```python
from build123d import *

# Parameters (mm, degrees)
FILLET1_R           = 6.35
SKETCH11_R          = 28.575
BOSS_EXTRUDE2_DEPTH = 1143
FILLET2_R           = 6.35
SCALE1_SCALE        = 0.5
SCALE2_SCALE        = 0.25


with BuildPart() as part:
    # Sketch7 → Revolve4 (revolve)
    with BuildSketch(Plane(origin=(0, 0, 0), x_dir=(1, 0, 0), z_dir=(0, 1, 0))):
        with BuildLine():
            Line((-190.055393274, 59.537811837), (0, 46.530218381))
            Line((0, 46.530218381), (0, 0))
            Line((0, 0), (-253.807316321, 0))
            ThreePointArc((-253.807316321, 0), (-234.86216044, 43.61495939), (-190.055393274, 59.537811837))
        make_face()
    revolve(axis=Axis((-253.807316321, 0, 0), (1, 0, 0)))

    # Fillet1
    fillet1_edges = [part.edges().sort_by_distance(p)[0] for p in [
        (0, 0, 46.530218381),
    ]]
    fillet(fillet1_edges, radius=FILLET1_R)

    # Sketch11 → Boss-Extrude2 (add)
    with BuildSketch(Plane(origin=(0, 0, 0), x_dir=(0, 0, -1), z_dir=(1, 0, 0))):
        Circle(SKETCH11_R)
    extrude(amount=BOSS_EXTRUDE2_DEPTH)

    # Sketch12 → Cut-Revolve1 (revolve, cut)
    with BuildSketch(Plane.XY):
        Polygon((0, 28.575), (1267.855525629, 6.186465308), (456.317793315, 229.960952638), align=None)
    revolve(axis=Axis((0, 0, 0), (1, 0, 0)), mode=Mode.SUBTRACT)

    # Fillet2
    fillet2_edges = [part.edges().sort_by_distance(p)[0] for p in [
        (1143, -8.391237232, 0),
    ]]
    fillet(fillet2_edges, radius=FILLET2_R)


with BuildPart() as part_1:
    # Scale1: scaled about (67.124128352, 0, 0)
    add(part.part.scale(SCALE1_SCALE).moved(Location((33.562064176, 0, 0))))


with BuildPart() as part_2:
    # Scale2: scaled about (67.124128352, 0, 0)
    add(part_1.part.scale(SCALE2_SCALE).moved(Location((50.343096264, 0, 0))))


solid = part_2.part
```
Source: CAD feature listing. Evaluate the final solid. Frame: model axes, mm. Coordinates: 2 decimals unless noted, no trailing zeros. Write each loop counter-clockwise with the first axis right and the second up, starting at its lowest first coordinate (ties: lowest second). Pieces come first, ordered by that corner, then holes. Notation, with made-up numbers: (78.25, 18.5) -> (115.25, 18.5) arc R8 cw to (115.25, 30.5) -> close; hole circle Ø2 at (26.5, 46). An arc over 180 degrees is marked (long way). Return JSON: item names as keys, results as strings. Group by question number.
1) Section query B-B, the plane x = 137.5. Return loops of the section in (y, z), plus the area to 3 significant figures.
2) Contact query for flat-ended pins moving along their axis: P1, Ø6, axis at x = 110, y = -1.5, coming from the +Z side; P2, Ø8, axis at x = 125, z = -1.5, coming from the +Y side; P3, Ø6, axis at x = 183.5, z = 3, coming from the -Y side. Output: stop coordinate, or through.
3) Section query A-A, the plane x = 86. Return loops of the section in (y, z), plus the area to 3 significant figures.
4) Ray query, line 1 along Z through (x, y) = (42, -1.5); line 2 along Z through (x, y) = (149, 1.75); line 3 along Y through (x, z) = (138, 1.5). Return the intervals inside material, ascending.
From the geometry:
{
 "1": {"outline": "circle Ø4.36 at (0, 0)", "area": "14.9 mm²"},
 "2": {"P1": "z = 2.71", "P2": "y = 2.47", "P3": "y = -1.38"},
 "3": {"outline": "circle Ø6.18 at (0, 0)", "area": "30.0 mm²"},
 "4": {"line 1": "-6.8 to 6.8", "line 2": "-0.92 to 0.92", "line 3": "-1.57 to 1.57"}
}
